Verification items for the finished model (mm, model axes). A direction names the side the tool comes from. Give positions to 0.01 mm unless a question says otherwise; leave off trailing zeros. Order: outer loops, then holes, each group sorted by start corner. A loop starts at its lowest first (then second) coordinate and runs counter-clockwise, first axis right, second up.
from build123d import *

# Parameters (mm, degrees)
SKETCH_1_W          = 64.5
SKETCH_1_H          = 70
EXTRUDE_1_DEPTH     = 20
FILLET_1_R          = 1
CUT_EXTRUDE_START   = 20
SKETCH_1_9_W        = 7.2
SKETCH_1_9_H        = 3.2
CUT_EXTRUDE_1_DEPTH = 2
EXTRUDE_START       = 18
SKETCH_1_10_W       = 3.5
SKETCH_1_10_H       = 3
EXTRUDE_2_DEPTH     = 2.5
SKETCH_2_R          = 2.5
CUT_EXTRUDE_2_DEPTH = 2


with BuildPart() as part:
    # 草图1 → 凸台-拉伸1 (new body)
    with BuildSketch(Plane(origin=(0, 0, 0), x_dir=(1, 0, 0), z_dir=(0, 1, 0))):
        Rectangle(SKETCH_1_W, SKETCH_1_H)
    extrude(amount=EXTRUDE_1_DEPTH)

    # 圆角1
    fillet_1_edges = [part.edges().sort_by_distance(p)[0] for p in [
        (0, 20, -35),
        (-32.25, 20, 0),
        (0, 20, 35),
        (-32.25, 0, 0),
        (0, 0, -35),
        (32.25, 0, 0),
        (0, 0, 35),
        (-32.25, 10, 35),
        (-32.25, 10, -35),
        (32.25, 10, -35),
        (32.25, 10, 35),
        (32.25, 20, 0),
    ]]
    fillet(fillet_1_edges, radius=FILLET_1_R)

    # 草图1<9> → 切除-拉伸1 (cut)
    with BuildSketch(Plane(origin=(0, 0, 0), x_dir=(1, 0, 0), z_dir=(0, 1, 0)).offset(CUT_EXTRUDE_START)):
        with Locations((19.75, 28.5)):
            Rectangle(SKETCH_1_9_W, SKETCH_1_9_H)
    extrude(amount=-CUT_EXTRUDE_1_DEPTH, mode=Mode.SUBTRACT)

    # 草图1<10> → 凸台-拉伸2 (add)
    with BuildSketch(Plane(origin=(0, 0, 0), x_dir=(1, 0, 0), z_dir=(0, 1, 0)).offset(EXTRUDE_START)):
        with Locations((18, 28.5)):
            Rectangle(SKETCH_1_10_W, SKETCH_1_10_H)
    extrude(amount=EXTRUDE_2_DEPTH)

    # 草图2 → 切除-拉伸2 (cut)
    with BuildSketch(Plane(origin=(0, 0, -35), x_dir=(-1, 0, 0), z_dir=(0, 0, -1))):
        with Locations((25.25, 15)):
            Circle(SKETCH_2_R)
    extrude(amount=-CUT_EXTRUDE_2_DEPTH, mode=Mode.SUBTRACT)


solid = part.part
(1) Go/stop test with flat-tipped pins: pin 1 (2.5 mm diameter, centred on x = -25.5, y = 14.5, fed in from -Z); pin 2 (19 mm diameter, centred on x = 9.5, z = -12.5, fed in from +Y); pin 3 (0.6 mm diameter, centred on x = 19.5, y = 19.5, fed in from -Z). Record where each tip stops, or that it passes through.
Solved:
pin 1: stops at z = -33
pin 2: stops at y = 20
pin 3: stops at z = -34.98
(2) Set-up check for faces 4 (the flat face through (20, 19, -30.1)), 5 (the cylindrical face through (-23.266, 13.479, -34.014)), 6 (the flat face through (32.25, 10, 0)): record each of +Z, -Z, +X, -X, +Y, -Y from which the full face is reachable in a straight line by a thin tool's end or side.
Solved:
face 4: +Y
face 5: -Z
face 6: +Z, -Z, +X, +Y, -Y
(3) Section check B-B, the plane x = -25.25. Enter the section's corners in (y, z), then the cut area to 3 significant figures.
Solved:
outline: (0, -34) arc R1 ccw to (1, -35) - (12.5, -35) - (12.5, -33) - (17.5, -33) - (17.5, -35) - (19, -35) arc R1 ccw to (20, -34) - (20, 34) arc R1 ccw to (19, 35) - (1, 35) arc R1 ccw to (0, 34) - close
area: 1,390 mm2
(4) Scan lines: line 1 (Y direction, x = -25.25, z = -34); line 2 (Y direction, x = 1, z = -4.5); line 3 (Y direction, x = -25.25, z = -34.5). Record each from-to range of solid material in increasing order.
Solved:
line 1: y = 0 to 12.5, 17.5 to 20
line 2: y = 0 to 20
line 3: y = 0.13 to 12.5, 17.5 to 19.87
(5) Section check C-C, the plane x = 9.5. Enter the section's corners in (y, z).
Solved:
outline: (0, -34) arc R1 ccw to (1, -35) - (19, -35) arc R1 ccw to (20, -34) - (20, 34) arc R1 ccw to (19, 35) - (1, 35) arc R1 ccw to (0, 34) - close
(6) Release check for a two-part mould opening along Z. For faces 1 (the flat face through (0, 0, 0)), 2 (the flat face through (20, 19, -26.9)), 3 (the flat face through (0, 10, -35)) record: pulls with the +Z half, pulls with the -Z half, needs draft (parallel to the pull), parting line crosses it, or undercut.
Solved:
face 1: needs draft
face 2: undercut
face 3: pulls with the -Z half
(7) Section check A-A, the plane z = -17.5. Enter the section's corners in (x, y).
Solved:
outline: (-32.25, 1) arc R1 ccw to (-31.25, 0) - (31.25, 0) arc R1 ccw to (32.25, 1) - (32.25, 19) arc R1 ccw to (31.25, 20) - (-31.25, 20) arc R1 ccw to (-32.25, 19) - close
